```python
from build123d import *

# Parameters (mm, degrees)
SKETCH1_R           = 4
BOSS_EXTRUDE1_DEPTH = 2
BOSS_EXTRUDE2_START = -2
SKETCH1_3_R         = 2
BOSS_EXTRUDE2_DEPTH = 9
BOSS_EXTRUDE3_START = -11
SKETCH1_4_R         = 4
BOSS_EXTRUDE3_DEPTH = 2
BOSS_EXTRUDE4_START = 3
BOSS_EXTRUDE4_DEPTH = 3
FILLET1_R           = 6
BOSS_EXTRUDE5_START = 3
BOSS_EXTRUDE5_DEPTH = 3
CIRPATTERN1_COUNT   = 6
CIRPATTERN1_ANGLE   = 34


with BuildPart() as part:
    # Sketch1 → Boss-Extrude1 (new body)
    with BuildSketch(Plane.YZ):
        with Locations(Location((0, 0, 0), (0, 0, 270))):
            Circle(SKETCH1_R)
    extrude(amount=-BOSS_EXTRUDE1_DEPTH)

    # Sketch1<3> → Boss-Extrude2 (add)
    with BuildSketch(Plane.YZ.offset(BOSS_EXTRUDE2_START)):
        with Locations(Location((0, 0, 0), (0, 0, 270))):
            Circle(SKETCH1_3_R)
    extrude(amount=-BOSS_EXTRUDE2_DEPTH)

    # Sketch1<4> → Boss-Extrude3 (add)
    with BuildSketch(Plane.YZ.offset(BOSS_EXTRUDE3_START)):
        with Locations(Location((0, 0, 0), (0, 0, 270))):
            Circle(SKETCH1_4_R)
    extrude(amount=-BOSS_EXTRUDE3_DEPTH)

    # Sketch2 → Boss-Extrude4 (add)
    with BuildSketch(Plane.YZ.offset(-11).offset(BOSS_EXTRUDE4_START)):
        with BuildLine():
            Line((2, 0), (2, 16))
            Line((2, 16), (-28.931042314, 26.795547064))
            ThreePointArc((-28.931042314, 26.795547064), (-29.786171027, 25.152339202), (-30.568468217, 23.473235781))
            ThreePointArc((-30.568468217, 23.473235781), (-33.95702666, 10.398285565), (-33.047270986, -3.077952637))
            Line((-33.047270986, -3.077952637), (-10.126725467, 5.61044016))
            ThreePointArc((-10.126725467, 5.61044016), (-4.591213765, 4.937628621), (-2, 0))
            ThreePointArc((-2, 0), (0, 2), (2, 0))
        make_face()
    extrude(amount=-BOSS_EXTRUDE4_DEPTH)

    # Fillet1
    fillet1_edges = [part.edges().sort_by_distance(p)[0] for p in [
        (-9.5, 2, 16),
    ]]
    fillet(fillet1_edges, radius=FILLET1_R)

    # Sketch2<3> → Boss-Extrude5 (add)
    with BuildSketch(Plane.YZ.offset(-11).offset(BOSS_EXTRUDE5_START)):
        with BuildLine():
            ThreePointArc((-30.568468217, 23.473235781), (-29.786171027, 25.152339202), (-28.931042314, 26.795547064))
            Line((-28.931042314, 26.795547064), (-32.992813147, 27.676701657))
            Line((-32.992813147, 27.676701657), (-33.441604676, 26.783065174))
            Line((-33.441604676, 26.783065174), (-30.568468217, 23.473235781))
        make_face()
    boss_extrude5 = extrude(amount=-BOSS_EXTRUDE5_DEPTH)

    # CirPattern1: Boss-Extrude5 ×6 about axis
    cirpattern1_axis = Axis((0, 8.12, 6.47), (1, 0, 0))
    for i in range(1, CIRPATTERN1_COUNT):
        add(boss_extrude5.rotate(cirpattern1_axis, i * CIRPATTERN1_ANGLE / (CIRPATTERN1_COUNT - 1)))


solid = part.part
```
Source: CAD feature listing. Evaluate the final solid. Frame: model axes, mm. A direction names the side the tool comes from. Give positions to 0.01 mm unless a question says otherwise; leave off trailing zeros. Loops run counter-clockwise (first coordinate to the right, second up) from the corner with the lowest first, then second, coordinate; pieces in that order, holes last. Notation, with made-up numbers: M 16.5,-24.5 L 59.5,-24.5 A12 cw 59.5,-7.5 Z; hole C -8,8.25 d9. An arc over 180 degrees is marked long. Put each result on its own line as item: value.
Q1. Pin query (flat end, axial travel): P1, Ø4, axis at x = -8, y = -24, coming from the -Z side; P2, Ø12, axis at y = -33.5, z = 21.5, coming from the -X side; P3, Ø9, axis at y = -25.5, z = 11, coming from the +X side. Return the tip coordinate at first contact, or that it passes through.
Response values:
P1: stops at z = -0.41
P2: stops at x = -11
P3: stops at x = -8
Q2. Mould query, pull axis Z, two halves, no side actions, for faces 4 (the flat face through (-9.479, -21.747, 1.205)), 5 (the flat face through (-11, -18, 13)), 6 (the cylindrical face through (-9.479, -34.018, 3.264)). Classes: released by +Z, released by -Z, zero draft, split by the parting line, or undercut.
Response values:
face 4: released by -Z
face 5: zero draft
face 6: undercut
Q3. Section B-B (y = 0). Return the cut outline in (x, z), and give its area (3 significant figures).
Response values:
outline: M -13,-4 L -11,-4 L -11,-2 L -2,-2 L -2,-4 L 0,-4 L 0,4 L -2,4 L -2,2 L -8,2 L -8,16.21 L -11,16.21 L -11,4 L -13,4 Z
area: 111 mm²
Q4. Section A-A (x = -4.75). Return the cut outline in (y, z), and give its area (3 significant figures).
Response values:
outline: C 0,0 d4
area: 12.6 mm²
Q5. Reachability of faces 1 (the flat face through (-9, 2, 6)), 2 (the cylindrical face through (-9.479, -30.824, 22.88)), 3 (the flat face through (-9.479, -35.292, 15.188)) from +Z, -Z, +X, -X, +Y, -Y: full face, straight path, thin tool, end or side. Return the list, or none.
Response values:
face 1: +Z, -Z, +Y
face 2: +X, -X
face 3: +X, -X, -Y
Q6. Line query: probe 1 along X at (y, z) = (-2, 1); probe 2 along X at (y, z) = (-7, 11); probe 3 along Z at (x, y) = (-8.75, -32). Output: solid intervals per line, ascending. Write a range as [from, to].
Response values:
probe 1: x = [-13, -8], [-2, 0]
probe 2: x = [-11, -8]
probe 3: z = [-2.68, 22.35], [25.12, 27.46]
Q7. Section C-C (z = 25). Return the cut outline in (x, y), and give its area (3 significant figures).
Response values:
outline: M -11,-31.89 L -8,-31.89 L -8,-23.79 L -11,-23.79 Z
area: 24.3 mm²
Q8. Section D-D (x = -11.5). Return the cut outline in (y, z).
Response values:
outline: C 0,0 d8
